```python
from build123d import *

# Parameters (mm, degrees)
SKETCH1_R           = 7.5
BOSS_EXTRUDE1_DEPTH = 3
SKETCH2_R           = 1.99
BOSS_EXTRUDE2_DEPTH = 26
CHAMFER1_SIZE       = 0.5
FILLET1_R           = 0.5


with BuildPart() as part:
    # Sketch1 → Boss-Extrude1 (new body)
    with BuildSketch(Plane.XY):
        Circle(SKETCH1_R)
    extrude(amount=BOSS_EXTRUDE1_DEPTH)

    # Sketch2 → Boss-Extrude2 (add)
    with BuildSketch(Plane.XY.offset(3)):
        with Locations(Location((0, 0, 0), (0, 0, 180))):
            Circle(SKETCH2_R)
    extrude(amount=BOSS_EXTRUDE2_DEPTH)

    # Chamfer1
    chamfer1_edges = [part.edges().sort_by_distance(p)[0] for p in [
        (1.99, 0, 29),
    ]]
    chamfer(chamfer1_edges, length=CHAMFER1_SIZE)

    # Fillet1
    fillet1_edges = [part.edges().sort_by_distance(p)[0] for p in [
        (1.99, 0, 3),
    ]]
    fillet(fillet1_edges, radius=FILLET1_R)


solid = part.part
```
The listing builds one solid part. Answer for the finished solid, in the listing's coordinates (mm). A direction names the side the tool comes from. Give positions to 0.01 mm unless a question says otherwise; leave off trailing zeros. Order: outer loops, then holes, each group sorted by start corner. A loop starts at its lowest first (then second) coordinate and runs counter-clockwise, first axis right, second up. Notation, with made-up numbers: (36.5, 27) - (68.5, 27) arc R23 ccw to (68.5, 61) - close; hole circle Ø5 at (-25.5, -6). An arc over 180 degrees is marked (long way). Answer in a Markdown table with one row per item. Add a question column.
Q1. Which of the six approach directions +Z, -Z, +X, -X, +Y, -Y give full straight-line access (tool end or side, diameter ignored) to faces 1 (the cylindrical face through (0.259, -1.973, 15.825)), 2 (the flat face through (0, 0, 0))?
Q2. The part is cut by section C-C (z = 6.5). Determine the outline of the cut face in (x, y), then the cut area to 3 significant figures.
Q3. The part is cut by section D-D (y = -4.5). Determine the outline of the cut face in (x, z), then the cut area to 3 significant figures.
Q4. Given P1, Ø3, axis at x = -4.5, y = 5, coming from the -Z side; P2, Ø8, axis at x = 1, z = 15, coming from the -Y side; P3, Ø3, axis at y = -1, z = 21.5, coming from the +X side; P4, Ø5, axis at x = 0.5, z = 14, coming from the +Y side, each flat-ended and moving along its own axis, determine where each tip first touches the part or whether it passes through.
Q5. The part is cut by section A-A (x = 0). Determine the outline of the cut face in (y, z).
Q6. Find the intervals of material crossed by line 1 along Z through (x, y) = (2.75, 4.25); line 2 along X through (y, z) = (-0.75, 18.75); line 3 along Y through (x, z) = (1.5, 16.5), in increasing order. Write a range as [from, to].
Determined:
| question | item | result |
|---|---|---|
| 1 | face 1 | +Z |
| 1 | face 2 | -Z, +X, -X, +Y, -Y |
| 2 | outline | circle Ø3.98 at (0, 0) |
| 2 | area | 12.4 mm² |
| 3 | outline | (-6, 0) - (6, 0) - (6, 3) - (-6, 3) - close |
| 3 | area | 36.0 mm² |
| 4 | P1 | stops at z = 0 |
| 4 | P2 | stops at y = -1.99 |
| 4 | P3 | stops at x = 1.99 |
| 4 | P4 | stops at y = 1.99 |
| 5 | outline | (-7.5, 0) - (7.5, 0) - (7.5, 3) - (2.49, 3) arc R0.5 cw to (1.99, 3.5) - (1.99, 28.5) - (1.49, 29) - (-1.49, 29) - (-1.99, 28.5) - (-1.99, 3.5) arc R0.5 cw to (-2.49, 3) - (-7.5, 3) - close |
| 6 | line 1 | z = [0, 3] |
| 6 | line 2 | x = [-1.84, 1.84] |
| 6 | line 3 | y = [-1.31, 1.31] |
